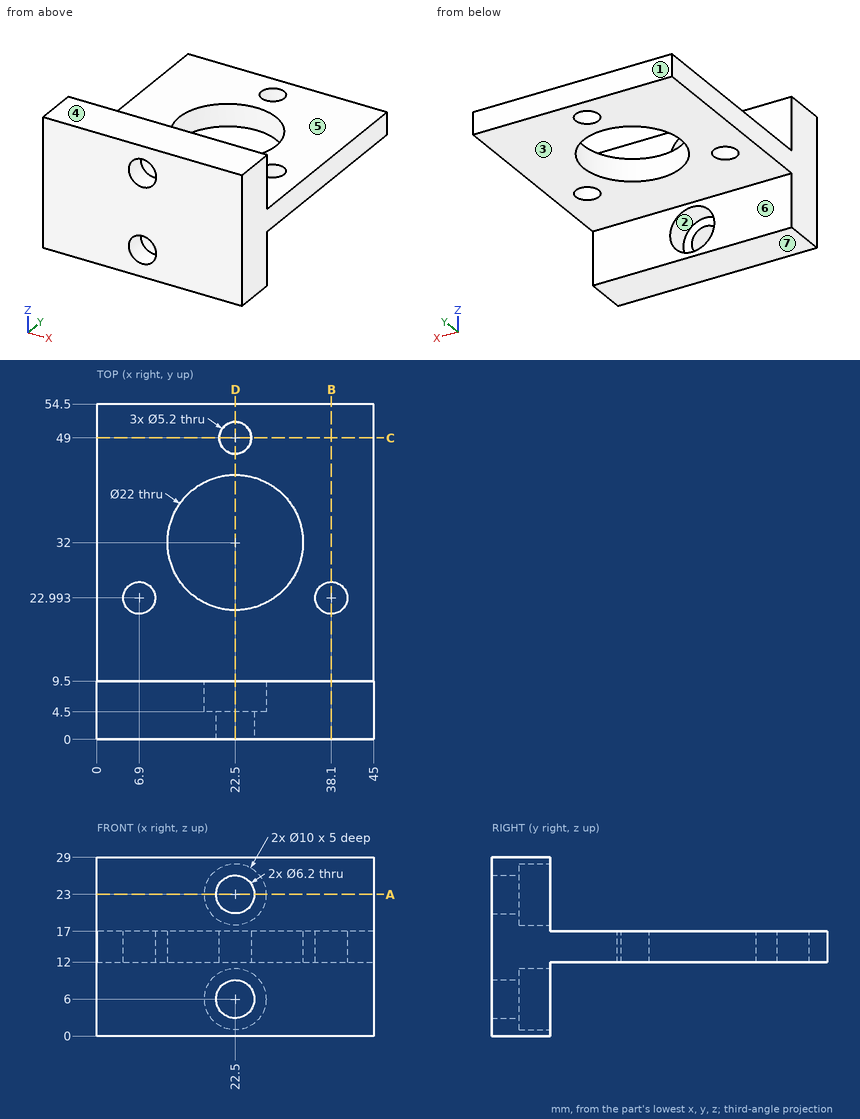
Part print with two shaded views. Sizes in mm from the minimum x, y, z corner. A direction names the side the tool comes from. Coordinates: 2 decimals unless noted, no trailing zeros. Write each loop counter-clockwise with the first axis right and the second up, starting at its lowest first coordinate (ties: lowest second). Pieces come first, ordered by that corner, then holes. Notation, with made-up numbers: M -19,18 L 29,18 A23 ccw 29,31 Z; hole C 44.25,78 d2. An arc over 180 degrees is marked long. Return JSON: item names as keys, results as strings.
Item 1: Slice it at A-A, the plane z = 23. Write the cut outline in (x, y), and give its area (3 significant figures).
Findings below:
{"outline": "M 0,0 L 19.4,0 L 19.4,4.5 L 17.5,4.5 L 17.5,9.5 L 0,9.5 Z; M 25.6,0 L 45,0 L 45,9.5 L 27.5,9.5 L 27.5,4.5 L 25.6,4.5 Z", "area": "350 mm2"}
Item 2: Drop flat-ended pins along their axis: pin 1 Ø4 at (x, y) = (6.9, 22.99) entering from -Z; pin 2 Ø8 at (x, z) = (22.5, 23) entering from +Y; pin 3 Ø12 at (x, y) = (15.5, 35) entering from +Z; pin 4 Ø8 at (x, z) = (23.5, 25) entering from +Y. Give the stop position or say it passes through.
Findings below:
{"pin 1": "passes through", "pin 2": "stops at y = 4.5", "pin 3": "stops at z = 17", "pin 4": "stops at y = 9.5"}
Item 3: Slice it at D-D, the plane x = 22.5. State how many separate pieces and enclosed holes the cut face has, and give its area (3 significant figures).
Findings below:
{"separate pieces": "5", "enclosed holes": "0", "area": "209 mm2"}
Item 4: Slice it at B-B, the plane x = 38.1. Write the cut outline in (y, z).
Findings below:
{"outline": "M 0,0 L 9.5,0 L 9.5,12 L 20.39,12 L 20.39,17 L 9.5,17 L 9.5,29 L 0,29 Z; M 25.59,12 L 54.5,12 L 54.5,17 L 25.59,17 Z"}
Item 5: Slice it at C-C, the plane y = 49. Write the cut outline in (x, z), and give its area (3 significant figures).
Findings below:
{"outline": "M 0,12 L 19.9,12 L 19.9,17 L 0,17 Z; M 25.1,12 L 45,12 L 45,17 L 25.1,17 Z", "area": "199 mm2"}
Item 6: Two-plate mould, pull along Z, no slides. Class the marked faces 1, 2, 3 and 4: +Z half, -Z half, draft (parallel to the pull), parting line (faces both ways), or undercut.
Findings below:
{"face 1": "draft", "face 2": "undercut", "face 3": "-Z half", "face 4": "+Z half"}
Item 7: Probe line 1 (Y direction, x = 22.5, z = 13.15); line 2 (Y direction, x = 6.9, z = 14.4); line 3 (Z direction, x = 20, y = 7). List the from-to ranges inside material, lowest first. Write a range as from..to.
Findings below:
{"line 1": "y = 0..21, 43..46.4, 51.6..54.5", "line 2": "y = 0..20.39, 25.59..54.5", "line 3": "z = 0..1.67, 10.33..18.67, 27.33..29"}
Item 8: Which spindle directions (+Z, -Z, +X, -X, +Y, -Y) get a long thin tool onto all of the face, cutting with end or side? Do the marked faces 5, 6 and 7. Say none if no direction does.
Findings below:
{"face 5": "+Z, +X, -X, +Y", "face 6": "-Z, +X, -X, +Y", "face 7": "-Z, +X, -X, +Y, -Y"}
